```python
from build123d import *

# Parameters (mm, degrees)
F1_DEPTH = 3
F2_R     = 1.5
F3_DEPTH = 5


with BuildPart() as f1:
    # F0 (on Top) → F1 (new body)
    with BuildSketch(Plane.XY):
        with BuildLine():
            Line((-7.5, 0), (-7.5, -2.783882))
            ThreePointArc((-7.5, -2.783882), (0, -8), (7.5, -2.783882))
            Line((7.5, -2.783882), (7.5, 0))
            Line((7.5, 0), (-7.5, 0))
        make_face()
    extrude(amount=F1_DEPTH)

    # F2 (on face) → F3 (cut)
    with BuildSketch(Plane(origin=(0, 0, 0), x_dir=(1, 0, 0), z_dir=(0, 0, -1))):
        with Locations((0, 2.783882)):
            Circle(F2_R)
    extrude(amount=-F3_DEPTH, mode=Mode.SUBTRACT)


solid = f1.part
```
Verification items for the finished model (mm, model axes). Round coordinates to 2 decimals unless told otherwise and drop trailing zeros. Write each loop counter-clockwise with the first axis right and the second up, starting at its lowest first coordinate (ties: lowest second). Pieces come first, ordered by that corner, then holes.
1. Section check D-D on x = 2. Enter the section's corners in (y, z).
2. Scan lines: L1, parallel to X at y = -3, z = 0.4; L2, parallel to Y at x = 1, z = 1.4; L3, parallel to X at y = -2.25, z = 2.75. Record each from-to range of solid material in increasing order.
3. Section check C-C on y = -6. Enter the section's corners in (x, z).
4. Section check A-A on x = 0. Enter the section's corners in (y, z).
5. Section check B-B on z = 2.55. Enter the section's corners in (x, y), plus the area to 3 significant figures.
6. Draft check along Y on faces 1 (the cylindrical face through (-0.33, -1.32, 1.48)), 2 (the flat face through (-7.5, -1, 1)), 3 (the cylindrical face through (0, -8, 1)). Enter one of: +Y half, -Y half, draft (parallel to the pull), parting line (faces both ways), or undercut.
Answer:
1. outline: (-7.75, 0) - (0, 0) - (0, 3) - (-7.75, 3) - close
2. L1: x = -7.42 to -1.48, 1.48 to 7.42
2. L2: y = -7.94 to -3.9, -1.67 to 0
2. L3: x = -7.5 to -1.4, 1.4 to 7.5
3. outline: (-5.29, 0) - (5.29, 0) - (5.29, 3) - (-5.29, 3) - close
4. outline: (-8, 0) - (-4.28, 0) - (-4.28, 3) - (-8, 3) - close; (-1.28, 0) - (0, 0) - (0, 3) - (-1.28, 3) - close
5. outline: (-7.5, -2.78) arc R8 ccw to (7.5, -2.78) - (7.5, 0) - (-7.5, 0) - close; hole circle Ø3 at (0, -2.78)
5. area: 91.6 mm2
6. face 1: undercut
6. face 2: draft
6. face 3: -Y half
